from build123d import *

# Parameters (mm, degrees)
SKETCH1_R           = 38.1
SKETCH1_R_2         = 6.35
BOSS_EXTRUDE1_DEPTH = 25.4
CUT_EXTRUDE1_DEPTH  = 19.05
SKETCH3_R           = 4.191
CUT_EXTRUDE2_DEPTH  = 135.408969451
FILLET1_R           = 7.62


with BuildPart() as part:
    # Sketch1 → Boss-Extrude1 (new body)
    with BuildSketch(Plane.XY):
        with BuildLine():
            Line((-18.576252895, 100.365223368), (19.281255226, 100.365223368))
            Line((19.281255226, 100.365223368), (19.281255226, 51.662487547))
            Line((19.281255226, 51.662487547), (85.717168685, 13.57632424))
            Line((85.717168685, 13.57632424), (54.8677317, -63.233808937))
            Line((54.8677317, -63.233808937), (31.764899533, -53.954963352))
            Line((31.764899533, -53.954963352), (12.667818141, -83.786038719))
            Line((12.667818141, -83.786038719), (-39.703691579, -83.786038719))
            Line((-39.703691579, -83.786038719), (-51.867045524, -14.691351221))
            ThreePointArc((-51.867045524, -14.691351221), (-52.552830667, 1.14672743), (-49.113541671, 16.622073237))
            Line((-49.113541671, 16.622073237), (-18.576252895, 100.365223368))
        make_face()
        Circle(SKETCH1_R, mode=Mode.SUBTRACT)
        with Locations((0, 87.665223368)):
            Circle(SKETCH1_R_2, mode=Mode.SUBTRACT)
        with Locations((-0.06167368, -71.086038719)):
            Circle(SKETCH1_R_2, mode=Mode.SUBTRACT)
        with Locations((-25.46167368, -71.075181752)):
            Circle(SKETCH1_R_2, mode=Mode.SUBTRACT)
    extrude(amount=BOSS_EXTRUDE1_DEPTH)

    # Sketch2 → Cut-Extrude1 (cut)
    with BuildSketch(Plane.XY):
        Polygon((54.8677317, -63.233808937), (31.764899533, -53.954963352), (66.538177491, 24.571193621), (85.717168685, 13.57632424), align=None)
    extrude(amount=CUT_EXTRUDE1_DEPTH, mode=Mode.SUBTRACT)

    # Sketch3 → Cut-Extrude2 (cut, through all)
    with BuildSketch(Plane.XY.offset(25.4)):
        with Locations((71.679164996, 8.361848351)):
            Circle(SKETCH3_R)
        with Locations((49.148937242, -47.734792738)):
            Circle(SKETCH3_R)
    extrude(amount=-CUT_EXTRUDE2_DEPTH, mode=Mode.SUBTRACT)

    # Fillet1
    fillet1_edges = [part.edges().sort_by_distance(p)[0] for p in [
        (12.667818141, -83.786038719, 12.7),
        (-39.703691579, -83.786038719, 12.7),
        (-18.576252895, 100.365223368, 12.7),
        (19.281255226, 100.365223368, 12.7),
        (19.281255226, 51.662487547, 12.7),
        (66.538177491, 24.571193621, 9.525),
    ]]
    fillet(fillet1_edges, radius=FILLET1_R)


solid = part.part
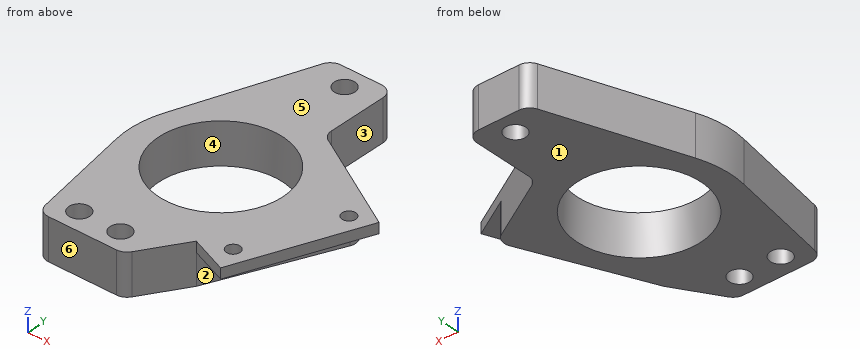
Verification items for the finished model (mm, model axes). Face numbers are marked on the shaded views. A direction names the side the tool comes from. Round coordinates to 2 decimals unless told otherwise and drop trailing zeros. Loops run counter-clockwise (first coordinate to the right, second up) from the corner with the lowest first, then second, coordinate; pieces in that order, holes last. Notation, with made-up numbers: (44.5, 73) - (90.5, 73) arc R24 ccw to (90.5, 89) - close; hole circle Ø4 at (61.5, -8). An arc over 180 degrees is marked (long way). Write item = value, one per line.
Q1. Sectioned sample at A-A on x = 0. Record the boundary of the cut face in (y, z), plus the area to 3 significant figures.
Here are the results:
outline = (-83.79, 0) - (-77.44, 0) - (-77.44, 25.4) - (-83.79, 25.4) - close; (-64.74, 0) - (-38.1, 0) - (-38.1, 25.4) - (-64.74, 25.4) - close; (38.1, 0) - (81.32, 0) - (81.32, 25.4) - (38.1, 25.4) - close; (94.02, 0) - (100.37, 0) - (100.37, 25.4) - (94.02, 25.4) - close
area = 2,100 mm^2
Q2. Material ranges on L1, parallel to Y at x = 0, z = 20.25; L2, parallel to Z at x = 50, y = -27; L3, parallel to Y at x = -8.5, z = 12.5, recorded low to high.
Here are the results:
L1 = -83.79 to -77.44, -64.74 to -38.1, 38.1 to 81.32, 94.02 to 100.37
L2 = 19.05 to 25.4
L3 = -83.79 to -37.14, 37.14 to 100.37
Q3. Sectioned sample at B-B on y = 31. Record the boundary of the cut face in (x, z).
Here are the results:
outline = (-43.87, 0) - (-22.15, 0) - (-22.15, 25.4) - (-43.87, 25.4) - close; (22.15, 0) - (55.32, 0) - (55.32, 25.4) - (22.15, 25.4) - close
Q4. Sectioned sample at D-D on y = -20. Record the boundary of the cut face in (x, z), plus the area to 3 significant figures.
Here are the results:
outline = (-50.93, 0) - (-32.43, 0) - (-32.43, 25.4) - (-50.93, 25.4) - close; (32.43, 0) - (46.8, 0) - (46.8, 19.05) - (72.23, 19.05) - (72.23, 25.4) - (32.43, 25.4) - close
area = 997 mm^2
Q5. Depth check by flat-ended pin: pin 1 (5 mm diameter, centred on x = 52.5, z = 11.5, fed in from +Y); pin 2 (5 mm diameter, centred on y = 75, z = 5, fed in from +X); pin 3 (10 mm diameter, centred on x = 23.5, z = 17.5, fed in from -Y). Enter the tip coordinate at first touch or a pass-through.
Here are the results:
pin_1 = 34.05
pin_2 = 19.28
pin_3 = -74.68
Q6. Tool access check on the marked faces 1, 2 and 3. Record the directions out of +Z, -Z, +X, -X, +Y, -Y that give a thin tool (end or side, any length) a straight path to the whole face; none if there is none.
Here are the results:
face_1 = -Z, +X, -X, +Y, -Y
face_2 = -Z, +X, -Y
face_3 = +Z, -Z, +X, +Y
Q7. Mould release check, pull along Y, two halves, no side actions. Record for the marked faces 4, 5 and 6: +Y half, -Y half, draft (parallel to the pull), parting line (faces both ways), or undercut.
Here are the results:
face_4 = undercut
face_5 = draft
face_6 = -Y half
Q8. Sectioned sample at C-C on z = 10.25. Record the boundary of the cut face in (x, y), plus the area to 3 significant figures.
Here are the results:
outline = (-51.87, -14.69) - (-40.81, -77.49) arc R7.62 ccw to (-33.31, -83.79) - (8.5, -83.79) arc R7.62 ccw to (14.92, -80.27) - (31.76, -53.95) - (63.76, 18.29) arc R7.62 ccw to (60.58, 27.99) - (23.11, 49.47) arc R7.62 cw to (19.28, 56.08) - (19.28, 92.75) arc R7.62 ccw to (11.66, 100.37) - (-13.24, 100.37) arc R7.62 ccw to (-20.4, 95.36) - (-49.11, 16.62) arc R60.69 ccw to start; hole circle Ø76.2 at (0, 0); hole circle Ø12.7 at (-25.46, -71.08); hole circle Ø12.7 at (-0.06, -71.09); hole circle Ø12.7 at (0, 87.67)
area = 9,270 mm^2
